Check sheet for the modelled part. Datum: model origin and axes. Units: mm. Face numbers are marked on the shaded views. Coordinates: 2 decimals unless noted, no trailing zeros. Use CSV: the item, a comma, the result in double quotes. Start each with the question number.
(1) Draft check along Z on the marked faces 1 and 2. Enter one of: pulls with the +Z half, pulls with the -Z half, needs draft (parallel to the pull), parting line crosses it, or undercut.
(2) Scan lines: line 1 (X direction, y = 8, z = 0.95); line 2 (Y direction, x = 17, z = 0.75). Record each from-to range of solid material in increasing order.
(3) Go/stop test with a flat-tipped pin: pin 1 Ø4 at (x, y) = (13, 3) entering from -Z. Record where the tip stops, or that it passes through.
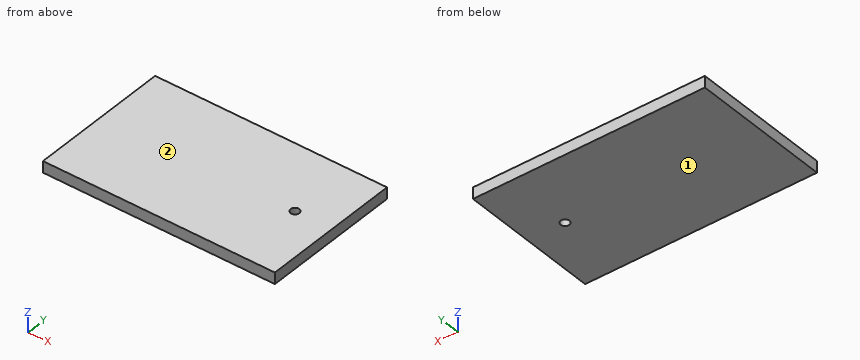
Autodesk Inventor part; units mm, degrees
ref_plane "YZ Plane" through (0, 0, 0) normal (1, 0, 0) x (0, 1, 0)
ref_plane "XZ Plane" through (0, 0, 0) normal (0, 1, 0) x (-1, 0, 0)
ref_plane "XY Plane" through (0, 0, 0) normal (0, 0, 1) x (1, 0, 0)
sketch "Sketch1" plane through (0, 0, 0) normal (0, 0, 1) x (1, 0, 0)
  line L0 (0, 14.001) -> (20.3353, 14.001)
  line L1 (20.3353, 14.001) -> (20.3353, 1.6382)
  line L2 (20.3353, 1.6382) -> (0, 1.6382)
  line L3 (0, 1.6382) -> (0, 14.001)
  point P0 (0, 0)
extrude "Extrusion1" add sketch "Sketch1" along normal blind 1
sketch "Sketch2" plane through (0, 0, 0) normal (0, 0, -1) x (-1, 0, 0)
  point P0 (0, 0)
sketch "Sketch3" plane through (0, 0, 0) normal (0, 0, -1) x (-1, 0, 0)
  point P0 (0, 0)
  point P1 (-17.0725, 7.955)
hole "Hole1" at (17.0725, 7.955, 0) direction (0, 0, 1) diameter 0.762 end through all
properties part number "1"
Outcome:
1,face 1,"pulls with the -Z half"
1,face 2,"pulls with the +Z half"
2,line 1,"x = 0 to 16.69, 17.45 to 20.34"
2,line 2,"y = 1.64 to 7.58, 8.33 to 14"
3,pin 1,"stops at z = 0"
